from build123d import *

# Parameters (mm, degrees)
F0_R     = 21
F0_R_2   = 12.5
F1_DEPTH = 40
F2_R     = 16
F3_DEPTH = 16
F4_R     = 16
F4_R_2   = 12.5
F5_DEPTH = 16
F6_SIZE  = 0.5


with BuildPart() as f1:
    # F0 (on Top) → F1 (new body)
    with BuildSketch(Plane.XY):
        Circle(F0_R)
        Circle(F0_R_2, mode=Mode.SUBTRACT)
    extrude(amount=F1_DEPTH)

    # F2 (on face) → F3 (cut)
    with BuildSketch(Plane.XY.offset(40)):
        Circle(F2_R)
    extrude(amount=-F3_DEPTH, mode=Mode.SUBTRACT)

    # F4 (on face) → F5 (cut)
    with BuildSketch(Plane(origin=(0, 0, 0), x_dir=(1, 0, 0), z_dir=(0, 0, -1))):
        Circle(F4_R)
        Circle(F4_R_2, mode=Mode.SUBTRACT)
    extrude(amount=-F5_DEPTH, mode=Mode.SUBTRACT)

    # F6
    f6_edges = [f1.edges().sort_by_distance(p)[0] for p in [
        (-21, 0, 0),
        (-16, 0, 0),
        (-21, 0, 40),
        (-16, 0, 40),
    ]]
    chamfer(f6_edges, length=F6_SIZE)


solid = f1.part
Design review of the part built by this model. Coordinates are the model's own, in mm. A direction names the side the tool comes from. Give positions to 0.01 mm unless a question says otherwise; leave off trailing zeros. Loops run counter-clockwise (first coordinate to the right, second up) from the corner with the lowest first, then second, coordinate; pieces in that order, holes last. Notation, with made-up numbers: (30, -1) - (57, -1) arc R8 cw to (57, 3) - close; hole circle Ø6 at (25, 53). An arc over 180 degrees is marked (long way). Write item = value, one per line.
1) Take a section at D-D on z = 19. State the section outline as (x, y) points, and give its area (3 significant figures).
Result sheet:
outline = circle Ø42 at (0, 0); hole circle Ø25 at (0, 0)
area = 895 mm2
2) Tool access review of faces 4 (the face through (-3.47, -15.62, 31.86)), 5 (the face through (-10, 8, 16)), 6 (the face through (1, 17, 0)): name each direction out of +Z, -Z, +X, -X, +Y, -Y from which nothing blocks a thin tool from reaching the whole face with its end or side.
Result sheet:
face_4 = +Z
face_5 = -Z
face_6 = -Z, +X, -X, +Y, -Y
3) Clearance check with flat-ended pins moving along their axes: pin 1 Ø5 at (x, z) = (6, 34) entering from -Y; pin 2 Ø10 at (x, z) = (7.5, 28.5) entering from +Y; pin 3 Ø8 at (x, y) = (0.5, 6) entering from -Z; pin 4 Ø6 at (y, z) = (1.5, 28.5) entering from +X. State where each tip first meets the part, or that it passes through.
Result sheet:
pin_1 = -20.71
pin_2 = 20.85
pin_3 = through
pin_4 = 21
4) Take a section at A-A on y = 0. State the section outline as (x, z) points.
Result sheet:
outline = (-21, 0.5) - (-20.5, 0) - (-16.5, 0) - (-16, 0.5) - (-16, 16) - (-12.5, 16) - (-12.5, 24) - (-16, 24) - (-16, 39.5) - (-16.5, 40) - (-20.5, 40) - (-21, 39.5) - close; (12.5, 16) - (16, 16) - (16, 0.5) - (16.5, 0) - (20.5, 0) - (21, 0.5) - (21, 39.5) - (20.5, 40) - (16.5, 40) - (16, 39.5) - (16, 24) - (12.5, 24) - close
5) Draft analysis for pull direction Y (two halves, no side actions). For faces 1 (the face through (1, 17, 40)), 2 (the face through (20.03, 6.31, 19.73)), 3 (the face through (11.923, 3.755, 19.944)), state which applies: +Y half, -Y half, draft (parallel to the pull), parting line (faces both ways), or undercut.
Result sheet:
face_1 = draft
face_2 = parting line
face_3 = undercut
6) To check wall thickness, follow line 1 (Y direction, x = 0, z = 6); line 2 (Y direction, x = 0, z = 22.5); line 3 (X direction, y = 13, z = 35). State the ranges of each line that lie inside material, in increasing order.
Result sheet:
line_1 = -21 to -16, 16 to 21
line_2 = -21 to -12.5, 12.5 to 21
line_3 = -16.49 to -9.33, 9.33 to 16.49
7) Take a section at C-C on z = 11. State the section outline as (x, y) points, and give its area (3 significant figures).
Result sheet:
outline = circle Ø42 at (0, 0); hole circle Ø32 at (0, 0)
area = 581 mm2
